For this review, take the finished solid that the model builds, in its own axes (mm). Face numbers are marked on the shaded views. Give positions to 0.01 mm unless a question says otherwise; leave off trailing zeros. Order: outer loops, then holes, each group sorted by start corner. A loop starts at its lowest first (then second) coordinate and runs counter-clockwise, first axis right, second up. Notation, with made-up numbers: (-40, -18.5) - (-24, -18.5) arc R18 ccw to (-24, -4.5) - close; hole circle Ø2 at (4.5, -18). An arc over 180 degrees is marked (long way). Answer as a JSON object with one key per item and string values. Group by question number.
from build123d import *

# Parameters (mm, degrees)
SKETCH_R            = 2.35
PAD_DEPTH           = 95
HOLE_D              = 3.4
HOLE_CBORE_D        = 6
HOLE_CBORE_DEPTH    = 3.4
HOLE001_D           = 3.4
HOLE001_CBORE_D     = 6
HOLE001_CBORE_DEPTH = 3.4
SKETCH003_R         = 2.6
SKETCH003_W         = 11.2
SKETCH003_H         = 9.2
POCKET_DEPTH        = 80.901
SKETCH004_W         = 13
SKETCH004_H         = 60.4
POCKET001_DEPTH     = 6.6


with BuildPart() as part:
    # Sketch → Pad (new body)
    with BuildSketch(Plane.XY):
        with BuildLine():
            Line((0, 0), (0, 65.9))
            ThreePointArc((15, 80.9), (4.393398, 76.506602), (0, 65.9))
            Line((15, 80.9), (47.9, 80.9))
            Line((47.9, 80.9), (47.9, 74.8998))
            ThreePointArc((46.0002, 73), (47.343561, 73.556439), (47.9, 74.8998))
            Line((46.0002, 73), (14.9999, 73))
            ThreePointArc((14.9999, 73), (9.979513, 70.920487), (7.9, 65.9001))
            Line((7.9, 65.9001), (7.9, 1.8998))
            ThreePointArc((6.0002, 0), (7.343561, 0.556439), (7.9, 1.8998))
            Line((6.0002, 0), (0, 0))
        make_face()
        with Locations((7.2218, 73.6782)):
            Circle(SKETCH_R, mode=Mode.SUBTRACT)
    extrude(amount=PAD_DEPTH)

    # Hole (through all)
    with Locations(Plane(origin=(0, 0, 0), x_dir=(0, -1, 0), z_dir=(-1, 0, 0))):
        with Locations((-6, 10), (-6, 85)):
            CounterBoreHole(HOLE_D / 2, HOLE_CBORE_D / 2, HOLE_CBORE_DEPTH)

    # Hole001 (through all)
    with Locations(Plane(origin=(0, 80.9, 0), x_dir=(-1, 0, 0), z_dir=(0, 1, 0))):
        with Locations((-42.9, 10), (-42.9, 85)):
            CounterBoreHole(HOLE001_D / 2, HOLE001_CBORE_D / 2, HOLE001_CBORE_DEPTH)

    # Sketch003 (on Face10 of Hole001) → Pocket (cut, through all)
    with BuildSketch(Plane(origin=(0, 80.9, 0), x_dir=(-1, 0, 0), z_dir=(0, 1, 0))):
        with Locations((-30.79, 58.76)):
            Circle(SKETCH003_R)
        with Locations((-30.79, 47.76)):
            Circle(SKETCH003_R)
        with BuildLine():
            Line((-31.31, 74.38), (-32.07, 74.38))
            ThreePointArc((-32.07, 74.38), (-32.989239, 73.999239), (-33.37, 73.08))
            Line((-33.37, 73.08), (-33.37, 66.48))
            ThreePointArc((-33.37, 66.48), (-32.989239, 65.560761), (-32.07, 65.18))
            Line((-32.07, 65.18), (-31.31, 65.18))
            ThreePointArc((-31.31, 65.18), (-30.390761, 65.560761), (-30.01, 66.48))
            Line((-30.01, 66.48), (-30.01, 73.08))
            ThreePointArc((-30.01, 73.08), (-30.390761, 73.999239), (-31.31, 74.38))
        make_face()
        with Locations((-27.79, 36.26)):
            Rectangle(SKETCH003_W, SKETCH003_H)
    extrude(amount=-POCKET_DEPTH, mode=Mode.SUBTRACT)

    # Sketch004 (on Face13 of Pocket) → Pocket001 (cut)
    with BuildSketch(Plane.XZ.offset(-73)):
        with Locations((28.5, 53.7)):
            Rectangle(SKETCH004_W, SKETCH004_H)
    extrude(amount=-POCKET001_DEPTH, mode=Mode.SUBTRACT)


solid = part.part
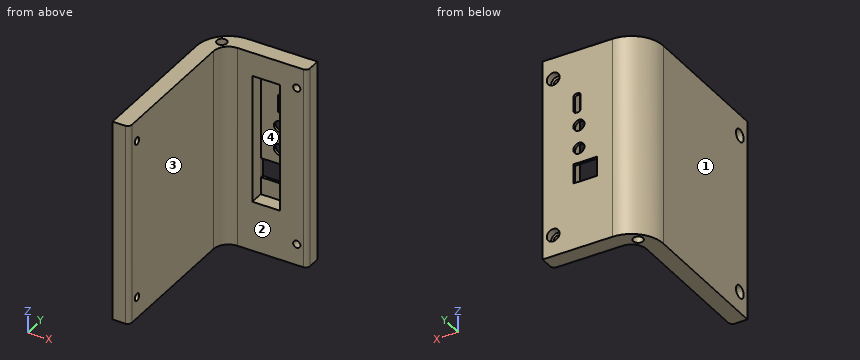
1) Consider section C-C (x = 42.9). Give the boundary of the cut face in (y, z).
2) For pin 1 (7 mm diameter, centred on x = 42.9, z = 85, fed in from -Y); pin 2 (5 mm diameter, centred on y = 36, z = 18.5, fed in from +X); pin 3 (3 mm diameter, centred on y = 7, z = 9, fed in from -X), all flat-tipped, find the tip position at first contact; note any pin that passes through.
3) For line 1 (Z direction, x = 0.7, y = 6); line 2 (X direction, y = 73.5, z = 40); line 3 (X direction, y = 59, z = 60), list the stretches that pass through material, from the lowest coordinate up.
4) Consider section A-A (z = 10). Give the boundary of the cut face in (x, y).
5) Consider section B-B (y = 6). Give the boundary of the cut face in (x, z).
6) Mouldability with a two-part tool opening along X and no side actions: class the marked faces 1, 2, 3 and 4 as released by +X, released by -X, zero draft, split by the parting line, or undercut.
7) Consider section D-D (z = 58.76). Give the boundary of the cut face in (x, y), plus the area to 3 significant figures.
Result set:
{
 "1": {"outline": "(73, 0) - (80.9, 0) - (80.9, 7) - (77.5, 7) - (77.5, 8.3) - (73, 8.3) - close; (73, 11.7) - (77.5, 11.7) - (77.5, 13) - (80.9, 13) - (80.9, 82) - (77.5, 82) - (77.5, 83.3) - (73, 83.3) - close; (73, 86.7) - (77.5, 86.7) - (77.5, 88) - (80.9, 88) - (80.9, 95) - (73, 95) - close"},
 "2": {"pin 1": "stops at y = 73", "pin 2": "stops at x = 7.9", "pin 3": "stops at x = 3.4"},
 "3": {"line 1": "z = 0 to 7, 13 to 82, 88 to 95", "line 2": "x = 2.07 to 4.88, 9.57 to 22, 35 to 47.28", "line 3": "x = 0 to 7.9"},
 "4": {"outline": "(0, 0) - (6, 0) arc R1.9 ccw to (7.9, 1.9) - (7.9, 4.3) - (3.4, 4.3) - (3.4, 3) - (0, 3) - close; (0, 9) - (3.4, 9) - (3.4, 7.7) - (7.9, 7.7) - (7.9, 65.9) arc R7.1 cw to (15, 73) - (41.2, 73) - (41.2, 77.5) - (39.9, 77.5) - (39.9, 80.9) - (15, 80.9) arc R15 ccw to (0, 65.9) - close; (44.6, 73) - (46, 73) arc R1.9 ccw to (47.9, 74.9) - (47.9, 80.9) - (45.9, 80.9) - (45.9, 77.5) - (44.6, 77.5) - close; hole circle Ø4.7 at (7.22, 73.68)"},
 "5": {"outline": "(0, 0) - (7.9, 0) - (7.9, 8.3) - (3.4, 8.3) - (3.4, 7) - (0, 7) - close; (0, 13) - (3.4, 13) - (3.4, 11.7) - (7.9, 11.7) - (7.9, 83.3) - (3.4, 83.3) - (3.4, 82) - (0, 82) - close; (0, 88) - (3.4, 88) - (3.4, 86.7) - (7.9, 86.7) - (7.9, 95) - (0, 95) - close"},
 "6": {"face 1": "released by -X", "face 2": "zero draft", "face 3": "released by +X", "face 4": "undercut"},
 "7": {"outline": "(0, 0) - (6, 0) arc R1.9 ccw to (7.9, 1.9) - (7.9, 65.9) arc R7.1 cw to (15, 73) - (22, 73) - (22, 79.6) - (28.19, 79.6) - (28.19, 80.9) - (15, 80.9) arc R15 ccw to (0, 65.9) - close; (33.39, 79.6) - (35, 79.6) - (35, 73) - (46, 73) arc R1.9 ccw to (47.9, 74.9) - (47.9, 80.9) - (33.39, 80.9) - close; hole circle Ø4.7 at (7.22, 73.68)", "area": "806 mm2"}
}
